Autodesk Inventor part; units mm, degrees
ref_plane "Work Plane2" through (1.75, 0, -1.5) normal (0, 0, 1) x (1, 0, 0)
ref_plane "YZ Plane" through (0, 0, 0) normal (1, 0, 0) x (0, 1, 0)
ref_plane "XZ Plane" through (0, 0, 0) normal (0, 1, 0) x (-1, 0, 0)
sketch "Sketch1" plane through (0, 0, 0) normal (0, 0, 1) x (1, 0, 0)
  line L0 (0, 0) -> (8.5, 0)
  line L1 (0, 0) -> (0, 1)
  line L2 (0, 1) -> (1.5, 1)
  line L3 (1.5, 1) -> (1.5, 1.5)
  line L4 (1.5, 1.5) -> (2, 1.5)
  line L5 (2, 1.5) -> (2, 3)
  line L6 (8.5, 0) -> (8.5, 8.9525) construction
  line L7 (2, 3) -> (8.5, 3)
  line L8 (17, 0) -> (8.5, 0)
  line L9 (17, 0) -> (17, 1)
  line L10 (17, 1) -> (15.5, 1)
  line L11 (15.5, 1) -> (15.5, 1.5)
  line L12 (15.5, 1.5) -> (15, 1.5)
  line L13 (15, 1.5) -> (15, 3)
  line L14 (15, 3) -> (8.5, 3)
  dimension "d0" = 7
  dimension "d1" = 1
  dimension "d2" = 1.5
  dimension "d3" = 1.5
  dimension "d4" = 3
  dimension "d5" = 0.5
revolve "Revolution1" add sketch "Sketch1" angle 360 about axis through (0, 0, 0) along (1, 0, 0)
ref_plane "Work Plane1" through (0.75, 0, 1) normal (0, 0, 1) x (1, 0, 0)
sketch "Sketch2" plane through (0.75, 0, 1) normal (0, 0, 1) x (1, 0, 0)
  line L0 (1.25, -3) -> (1.25, 3)
  line L1 (14.25, -3) -> (14.25, 3)
  line L2 (0.75, -1.5) -> (0.75, 1.5)
  line L3 (1.25, -1.5) -> (1.25, 1.5)
  line L4 (14.25, -1.5) -> (14.25, 1.5)
  line L5 (14.75, -1.5) -> (14.75, 1.5)
  line L6 (0.75, 1.5) -> (1.25, 1.5)
  line L7 (0.75, -1.5) -> (1.25, -1.5)
  line L8 (14.25, 1.5) -> (14.75, 1.5)
  line L9 (14.25, -1.5) -> (14.75, -1.5)
  line L10 (1.25, -3) -> (14.25, -3)
  line L11 (1.25, 3) -> (14.25, 3)
  point P0 (-0.75, 0)
extrude "Extrusion1" cut sketch "Sketch2" along normal through all
ref_plane "Work Plane2" through (1.75, 0, -1.5) normal (0, 0, 1) x (1, 0, 0)
sketch "Sketch3" plane through (1.75, 0, -1.5) normal (0, 0, 1) x (1, 0, 0)
  line L0 (0.25, 3) -> (13.25, 3)
  line L1 (13.25, -3) -> (13.25, 3)
  line L2 (0.25, -3) -> (0.25, 3)
  line L3 (0.25, -3) -> (13.25, -3)
  point P0 (-1.75, 0)
  point P1 (13.25, -2.8284)
  point P2 (13.25, 2.8284)
  point P3 (0.25, -2.8284)
  point P4 (0.25, 2.8284)
extrude "Extrusion2" cut sketch "Sketch3" against normal through all
sketch "Sketch4" plane through (1.75, 0, -1.5) normal (0, 0, 1) x (1, 0, 0)
  line L0 (15.25, -1) -> (15.25, 1)
  line L1 (15.25, 0) -> (-1.75, 0) construction
  line L2 (6.75, 0) -> (6.75, 2.8511) construction
  line L3 (-1.75, 0) -> (15.25, 0) construction
  point P0 (10.75, 0)
  point P1 (2.75, 0)
  dimension "d11" = 8
hole "Hole1" at (12.5, 0, -1.5) at (4.5, 0, -1.5) direction (0, 0, 1) diameter 2 end through all counterbore diameter 4 counterbore depth 2
equation "\"d0\" = 0.5 * finger_inner_width"
equation "\"d4\" = 0.5 * finger_shaft_diameter"
equation "\"finger_mounting_screw_distance\" = 8"
equation "\"finger_shaft_diameter\" = 6"
equation "\"finger_inner_width\" = 14"
properties part number "0th_finger_mount"
Model file for the job. Use its own axes, mm. A direction names the side the tool comes from. Coordinates: 2 decimals unless noted, no trailing zeros. Order: outer loops, then holes, each group sorted by start corner. A loop starts at its lowest first (then second) coordinate and runs counter-clockwise, first axis right, second up. Notation, with made-up numbers: M 50.25,-14.5 L 94.25,-14.5 A9 ccw 94.25,-2.5 Z; hole C 62.5,42 d8. An arc over 180 degrees is marked long. Return JSON: item names as keys, results as strings.
1. Saw through at A-A (x = 12.5). Give the cut face in (y, z).
Ans:
{"outline": "M -2.83,1 A3 ccw -2.6,-1.5 L -2,-1.5 L -2,0.5 L -1,0.5 L -1,1 Z; M 1,0.5 L 2,0.5 L 2,-1.5 L 2.6,-1.5 A3 ccw 2.83,1 L 1,1 Z"}
2. Flat gauge pins, fed straight in: pin 1 (1 mm diameter, centred on x = 8.5, z = -1, fed in from +Y); pin 2 (1.2 mm diameter, centred on x = 5, y = 0.5, fed in from -Z); pin 3 (0.8 mm diameter, centred on y = -1.5, z = 0.5, fed in from +X). Where does each tip first touch, or does it go through?
Ans:
{"pin 1": "y = 2.96", "pin 2": "z = 0.5", "pin 3": "x = 15.5"}
3. Tool access for faces 5 (the face through (10.517, -0.26, -0.486)), 6 (the face through (15.5, -0.4, -1.1)), 7 (the face through (1, 0, -1)): list every direction of +Z, -Z, +X, -X, +Y, -Y with a clear straight run to the whole face (end or side of a thin tool).
Ans:
{"face 5": "-Z", "face 6": "+X", "face 7": "-X"}
4. Saw through at B-B (z = 0). Give the cut face in (x, y), and give its area (3 significant figures).
Ans:
{"outline": "M 0,-1 L 1.5,-1 L 1.5,-1.5 L 2,-1.5 L 2,-3 L 15,-3 L 15,-1.5 L 15.5,-1.5 L 15.5,-1 L 17,-1 L 17,1 L 15.5,1 L 15.5,1.5 L 15,1.5 L 15,3 L 2,3 L 2,1.5 L 1.5,1.5 L 1.5,1 L 0,1 Z; hole C 4.5,0 d4; hole C 12.5,0 d4", "area": "61.9 mm^2"}
5. Saw through at C-C (y = -0.5). Give the number of separate pieces and of enclosed holes in the cut face, and give its area (3 significant figures).
Ans:
{"separate pieces": "3", "enclosed holes": "0", "area": "22.9 mm^2"}
6. Saw through at D-D (y = -1.75). Give the cut face in (x, z), and give its area (3 significant figures).
Ans:
{"outline": "M 2,-1.5 L 3.53,-1.5 L 3.53,0.5 L 5.47,0.5 L 5.47,-1.5 L 11.53,-1.5 L 11.53,0.5 L 13.47,0.5 L 13.47,-1.5 L 15,-1.5 L 15,1 L 2,1 Z", "area": "24.8 mm^2"}
7. Drill centre lines: probe 1 along X at (y, z) = (0, 0.7); probe 2 along X at (y, z) = (0, 0.1); probe 3 along X at (y, z) = (-2.25, 0.8). Where is each one in solid material? Low to high.
Ans:
{"probe 1": "0 to 3.5, 5.5 to 11.5, 13.5 to 17", "probe 2": "0 to 2.5, 6.5 to 10.5, 14.5 to 17", "probe 3": "2 to 15"}
8. Pull direction X, two halves, no side cores. Call faces 1 (the face through (15, 2, 0)), 2 (the face through (0, 0, 0)), 3 (the face through (6.452, -0.434, -0.486)), 4 (the face through (1.8, 0, -1.5)): +X half, -X half, draft (parallel to the pull), parting line (faces both ways), or undercut.
Ans:
{"face 1": "+X half", "face 2": "-X half", "face 3": "undercut", "face 4": "draft"}
